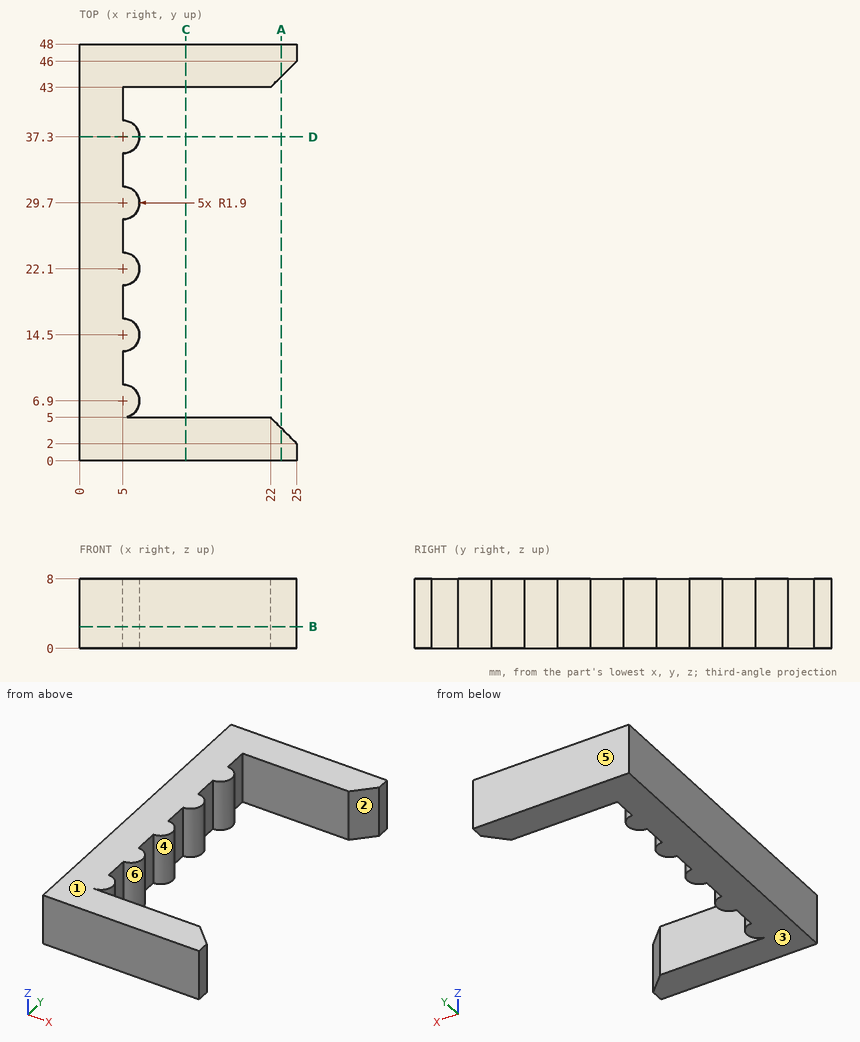
Answer from the drawing. Dimensions are ordinates in mm from the lowest x, y and z of the part. A direction names the side the tool comes from. Coordinates: 2 decimals unless noted, no trailing zeros. Loops run counter-clockwise (first coordinate to the right, second up) from the corner with the lowest first, then second, coordinate; pieces in that order, holes last.
1) Section B-B (z = 2.5) is taken. Give the vertices of the cut face in (x, y).
Results:
outline: (0, 0) - (25, 0) - (25, 2) - (22, 5) - (5, 5) arc R1.9 ccw to (5, 8.8) - (5, 12.6) arc R1.9 ccw to (5, 16.4) - (5, 20.2) arc R1.9 ccw to (5, 24) - (5, 27.8) arc R1.9 ccw to (5, 31.6) - (5, 35.4) arc R1.9 ccw to (5, 39.2) - (5, 43) - (22, 43) - (25, 46) - (25, 48) - (0, 48) - close
2) Flat-ended cylindrical pins translate along their axes: pin 1 (3 mm diameter, centred on y = 32.5, z = 4.5, fed in from +X); pin 2 (1.1 mm diameter, centred on y = 42, z = 5, fed in from +X); pin 3 (4 mm diameter, centred on y = 26.5, z = 5, fed in from +X). Find the tip coordinate at first contact, or state that the pin passes through.
Results:
pin 1: stops at x = 6.39
pin 2: stops at x = 5
pin 3: stops at x = 6.47
3) For a pull along Y with two mould halves and no side action, classify the marked faces 3, 4, 5 and 6 as +Y half, -Y half, draft (parallel to the pull), parting line (faces both ways), or undercut.
Results:
face 3: draft
face 4: undercut
face 5: +Y half
face 6: undercut
4) Section C-C (x = 12.25) is taken. Give the vertices of the cut face in (y, z).
Results:
outline: (0, 0) - (5, 0) - (5, 8) - (0, 8) - close; (43, 0) - (48, 0) - (48, 8) - (43, 8) - close
5) Consider probe 1 along Y at (x, z) = (12, 4.5); probe 2 along X at (y, z) = (42, 5.25); probe 3 along Y at (x, z) = (23.5, 4.25). Determine where each line is inside the solid, lowest interval first.
Results:
probe 1: y = 0 to 5, 43 to 48
probe 2: x = 0 to 5
probe 3: y = 0 to 3.5, 44.5 to 48
6) For the marked faces 1 and 2, determine the directions among +Z, -Z, +X, -X, +Y, -Y from which every point of the face is accessible in a straight line to the end or side of a thin tool.
Results:
face 1: +Z, +X, -X, +Y, -Y
face 2: +Z, -Z, +X
7) Section D-D (y = 37.3) is taken. Give the vertices of the cut face in (x, z).
Results:
outline: (0, 0) - (6.9, 0) - (6.9, 8) - (0, 8) - close
8) Section A-A (x = 23.25) is taken. Give the vertices of the cut face in (y, z), plus the area to 3 significant figures.
Results:
outline: (0, 0) - (3.75, 0) - (3.75, 8) - (0, 8) - close; (44.25, 0) - (48, 0) - (48, 8) - (44.25, 8) - close
area: 60.0 mm2
